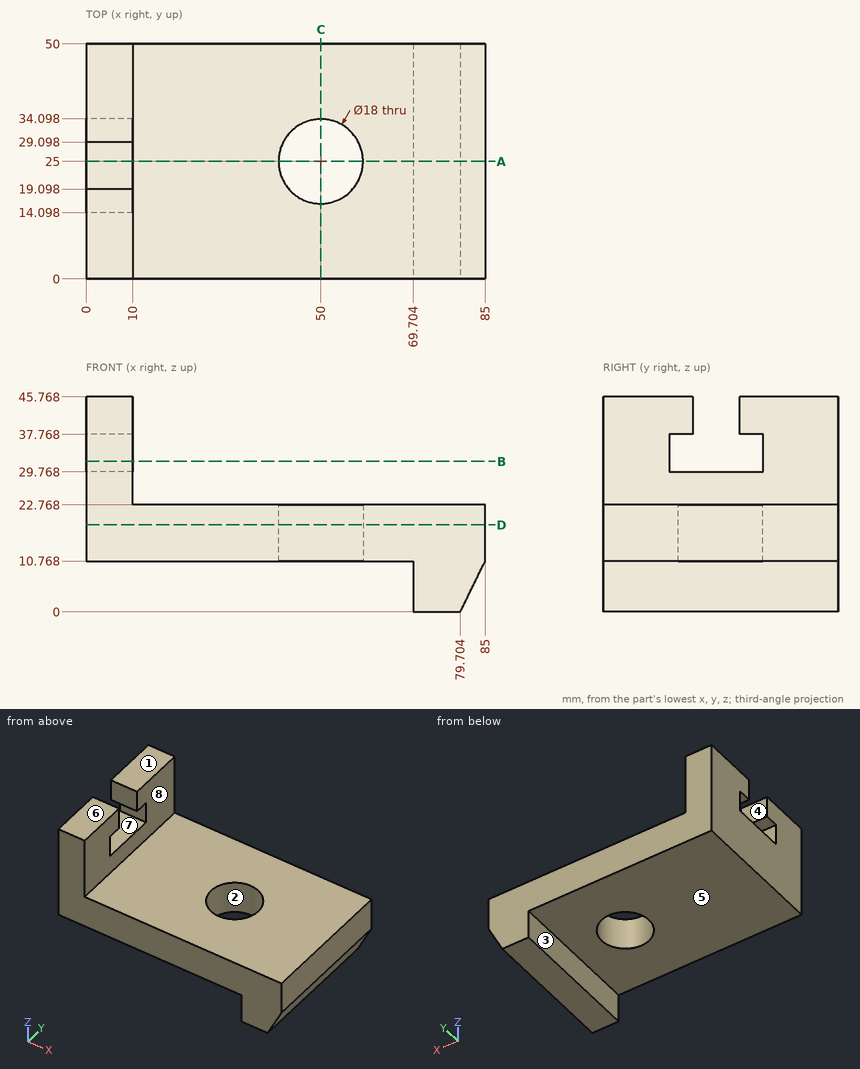
Can you work these out from the drawing? Everything is in mm from the part's minimum corner. A direction names the side the tool comes from. Round coordinates to 2 decimals unless told otherwise and drop trailing zeros. Write each loop counter-clockwise with the first axis right and the second up, starting at its lowest first coordinate (ties: lowest second). Pieces come first, ordered by that corner, then holes. Notation, with made-up numbers: (57, 39.25) - (75, 39.25) arc R21 cw to (75, 59.25) - close; hole circle Ø4 at (83, -0.75). An arc over 180 degrees is marked (long way). Write each question's results on one line, items separated by ' | '. Start each with the question number.
1) Suppose I cut it at C-C (x = 50). List the corners of the cut face in (y, z) for me, and give its area (3 significant figures).
2) For pin 1 Ø2.5 at (x, z) = (7, 36) entering from -Y; pin 2 Ø10 at (x, y) = (69.5, 25.5) entering from +Z; pin 3 Ø4 at (x, y) = (61, 30.5) entering from -Z; pin 4 Ø11 at (x, y) = (50, 25) entering from +Z (1 decimal), each with a flat end and sliding along its axis, tell me the tip position at first contact or that it passes through.
3) Suppose I cut it at D-D (z = 18.5). List the corners of the cut face in (x, y) for me, and give its area (3 significant figures).
4) We'd pull the mould along X, two halves only. Please class the marked faces 1, 2 and 3: released by +X, released by -X, zero draft, split by the parting line, or undercut.
5) Which directions (+Z, -Z, +X, -X, +Y, -Y) give clear straight access to the entire face, cutting with the end or side of a thin tool? Please do the marked faces 4, 5, 6, 7 and 8.
6) Please list where these lines run through material, in increasing order: line 1 (Y direction, x = 50, z = 16); line 2 (X direction, y = 32, z = 39); line 3 (Z direction, x = 14, y = 47).
7) Suppose I cut it at B-B (z = 32). List the corners of the cut face in (x, y) for me.
8) Suppose I cut it at A-A (y = 25). List the corners of the cut face in (x, z) for me, and give its area (3 significant figures).
Here are the results:
1) outline: (0, 10.77) - (16, 10.77) - (16, 22.77) - (0, 22.77) - close; (34, 10.77) - (50, 10.77) - (50, 22.77) - (34, 22.77) - close | area: 384 mm2
2) pin 1: stops at y = 0 | pin 2: stops at z = 22.77 | pin 3: stops at z = 10.77 | pin 4: passes through
3) outline: (0, 0) - (85, 0) - (85, 50) - (0, 50) - close; hole circle Ø18 at (50, 25) | area: 4,000 mm2
4) face 1: zero draft | face 2: undercut | face 3: released by -X
5) face 4: +Z, +X, -X | face 5: -Z, -X, +Y, -Y | face 6: +Z, +X, -X, +Y, -Y | face 7: +X, -X | face 8: +Z, +X, +Y, -Y
6) line 1: y = 0 to 16, 34 to 50 | line 2: x = 0 to 10 | line 3: z = 10.77 to 22.77
7) outline: (0, 0) - (10, 0) - (10, 14.1) - (0, 14.1) - close; (0, 34.1) - (10, 34.1) - (10, 50) - (0, 50) - close
8) outline: (0, 10.77) - (41, 10.77) - (41, 22.77) - (10, 22.77) - (10, 29.77) - (0, 29.77) - close; (59, 10.77) - (69.7, 10.77) - (69.7, 0) - (79.7, 0) - (85, 10.77) - (85, 22.77) - (59, 22.77) - close | area: 1,010 mm2
